from build123d import *

# Parameters (mm, degrees)
BOSS_EXTRUDE2_DEPTH = 33
CUT_EXTRUDE1_DEPTH  = 28
SKETCH3_R           = 10
CUT_EXTRUDE2_DEPTH  = 6
SKETCH5_R           = 2.9
BOSS_EXTRUDE3_DEPTH = 28.7
CIRPATTERN1_COUNT   = 3
SKETCH6_R           = 1
BOSS_EXTRUDE4_DEPTH = 2


with BuildPart() as part:
    # Sketch1 → Boss-Extrude2 (new body)
    with BuildSketch(Plane(origin=(0, 0, 0), x_dir=(1, 0, 0), z_dir=(0, 1, 0))):
        with BuildLine():
            Line((68.783761953, -39.4), (157.583761953, -39.4))
            ThreePointArc((157.583761953, -39.4), (164.654829765, -36.471067812), (167.583761953, -29.4))
            Line((167.583761953, -29.4), (167.583761953, 29.4))
            ThreePointArc((167.583761953, 29.4), (164.654829765, 36.471067812), (157.583761953, 39.4))
            Line((157.583761953, 39.4), (68.783761953, 39.4))
            ThreePointArc((68.783761953, 39.4), (61.283761953, 46.9), (53.783761953, 39.4))
            Line((53.783761953, 39.4), (30.783761953, 39.4))
            ThreePointArc((30.783761953, 39.4), (21.761629353, 45.015902611), (11.75641742, 48.598216525))
            ThreePointArc((11.75641742, 48.598216525), (10.817431593, 49.174777372), (10.394956543, 50.192437248))
            Line((10.394956543, 50.192437248), (8.132117785, 78.35566571))
            ThreePointArc((8.132117785, 78.35566571), (7.562644675, 79.526094921), (6.350366597, 80))
            Line((6.350366597, 80), (-6.350366597, 80))
            ThreePointArc((-6.350366597, 80), (-7.562644675, 79.526094921), (-8.132117785, 78.35566571))
            Line((-8.132117785, 78.35566571), (-10.394956543, 50.192437248))
            ThreePointArc((-10.394956543, 50.192437248), (-10.817431593, 49.174777372), (-11.75641742, 48.598216525))
            ThreePointArc((-11.75641742, 48.598216525), (-50, 0), (-11.75641742, -48.598216525))
            ThreePointArc((-11.75641742, -48.598216525), (-10.817431593, -49.174777372), (-10.394956543, -50.192437248))
            Line((-10.394956543, -50.192437248), (-8.132117785, -78.35566571))
            ThreePointArc((-8.132117785, -78.35566571), (-7.562644675, -79.526094921), (-6.350366597, -80))
            Line((-6.350366597, -80), (6.350366597, -80))
            ThreePointArc((6.350366597, -80), (7.562644675, -79.526094921), (8.132117785, -78.35566571))
            Line((8.132117785, -78.35566571), (10.394956543, -50.192437248))
            ThreePointArc((10.394956543, -50.192437248), (10.817431593, -49.174777372), (11.75641742, -48.598216525))
            ThreePointArc((11.75641742, -48.598216525), (21.761629353, -45.015902611), (30.783761953, -39.4))
            Line((30.783761953, -39.4), (53.783761953, -39.4))
            ThreePointArc((53.783761953, -39.4), (61.283761953, -46.9), (68.783761953, -39.4))
        make_face()
    extrude(amount=BOSS_EXTRUDE2_DEPTH)

    # Sketch2 → Cut-Extrude1 (cut)
    with BuildSketch(Plane(origin=(0, 33, 0), x_dir=(1, 0, 0), z_dir=(0, 1, 0))):
        with BuildLine():
            Line((23.583761953, 29.4), (23.583761953, -29.4))
            ThreePointArc((23.583761953, -29.4), (25.702607781, -35.555274886), (31.161243737, -39.102134069))
            ThreePointArc((31.161243737, -39.102134069), (22.770762082, -44.513957297), (13.472291615, -48.150777342))
            Line((13.472291615, -48.150777342), (13.472291615, -85.250601705))
            Line((13.472291615, -85.250601705), (-13.472291615, -85.250601705))
            Line((-13.472291615, -85.250601705), (-13.472291615, -48.150777342))
            ThreePointArc((-13.472291615, -48.150777342), (-50, 0), (-13.472291615, 48.150777342))
            Line((-13.472291615, 48.150777342), (-13.472291615, 85.250601705))
            Line((-13.472291615, 85.250601705), (13.472291615, 85.250601705))
            Line((13.472291615, 85.250601705), (13.472291615, 48.150777342))
            ThreePointArc((13.472291615, 48.150777342), (22.770762082, 44.513957297), (31.161243737, 39.102134069))
            ThreePointArc((31.161243737, 39.102134069), (25.702607781, 35.555274886), (23.583761953, 29.4))
        make_face()
    extrude(amount=-CUT_EXTRUDE1_DEPTH, mode=Mode.SUBTRACT)

    # Sketch3 → Cut-Extrude2 (cut, through all)
    with BuildSketch(Plane(origin=(0, 5, 0), x_dir=(1, 0, 0), z_dir=(0, 1, 0))):
        Circle(SKETCH3_R)
    extrude(amount=-CUT_EXTRUDE2_DEPTH, mode=Mode.SUBTRACT)

    # Sketch5 → Boss-Extrude3 (add)
    with BuildSketch(Plane(origin=(0, 5, 0), x_dir=(1, 0, 0), z_dir=(0, 1, 0))):
        with Locations((-34.9, 0)):
            Circle(SKETCH5_R)
    boss_extrude3 = extrude(amount=BOSS_EXTRUDE3_DEPTH)

    # CirPattern1: Boss-Extrude3 ×3 about axis
    cirpattern1_axis = Axis((0, 0, 0), (0, 1, 0))
    for i in range(1, CIRPATTERN1_COUNT):
        add(boss_extrude3.rotate(cirpattern1_axis, i * 360 / CIRPATTERN1_COUNT))

    # Sketch6 → Boss-Extrude4 (add)
    with BuildSketch(Plane(origin=(0, 5, 0), x_dir=(1, 0, 0), z_dir=(0, 1, 0))):
        with Locations((-17.896238047, -8.587616886)):
            Circle(SKETCH6_R)
    extrude(amount=BOSS_EXTRUDE4_DEPTH)


solid = part.part
Part model, mm, in its own coordinate system. A direction names the side the tool comes from. Coordinates: 2 decimals unless noted, no trailing zeros. Loops run counter-clockwise (first coordinate to the right, second up) from the corner with the lowest first, then second, coordinate; pieces in that order, holes last. Notation, with made-up numbers: M 38,64 L 84,64 A11 ccw 84,70 Z; hole C 82,-0.5 d7. An arc over 180 degrees is marked long. Use a Markdown table: item, result. Add a question column.
Q1. Which spindle directions (+Z, -Z, +X, -X, +Y, -Y) get a long thin tool onto all of the face, cutting with end or side? Do faces 1 (the cylindrical face through (15.31, 19.15, -32.18)), 2 (the flat face through (95, 33, -1)), 3 (the flat face through (113, 16, 39.4)), 4 (the flat face through (0, 2, 80)), 5 (the flat face through (114, 16, -39.4)). Say none if no direction does.
Q2. Cut at B-B (z = 0). Write the cut outline in (x, y), and give its area (3 significant figures).
Q3. Cut at A-A (x = 0). Write the cut outline in (y, z), and give its area (3 significant figures).
Q4. Cut at C-C (y = 12). Write the cut outline in (x, z).
Q5. Cut at D-D (x = 26.5). Write the cut outline in (y, z).
Q6. Probe L1, parallel to Z at x = 0, y = 2.1; L2, parallel to X at y = 2.8, z = 0; L3, parallel to Z at x = 151, y = 19. List the from-to ranges inside material, lowest first.
Q7. Mould opens along X. For faces 6 (the flat face through (167.584, 16, 0)), 7 (the flat face through (18, 33.7, -30)), 8 (the cylindrical face through (-32.134, 19.149, -0.871)) say: +X half, -X half, draft (parallel to the pull), parting line (faces both ways), or undercut.
Q8. Pin check, flat tips, straight feed: P1, Ø11.5, axis at x = 40.5, y = 24.5, coming from the +Z side; P2, Ø10, axis at y = 19.5, z = 36, coming from the -X side; P3, Ø0.6, axis at x = -18, z = 8, coming from the +Y side; P4, Ø1.5, axis at y = 11.5, z = 49.5, coming from the +X side. Stop position of each tip, or through.
Worked out:
| question | item | result |
|---|---|---|
| 1 | face 1 | +Y |
| 1 | face 2 | +Z, -Z, +X, +Y |
| 1 | face 3 | +Z, +X, +Y, -Y |
| 1 | face 4 | +Z, +X, -X, +Y, -Y |
| 1 | face 5 | -Z, +X, +Y, -Y |
| 2 | outline | M -50,0 L -10,0 L -10,5 L -32,5 L -32,33.7 L -37.8,33.7 L -37.8,5 L -50,5 Z; M 10,0 L 167.58,0 L 167.58,33 L 23.58,33 L 23.58,5 L 10,5 Z |
| 2 | area | 5,190 mm2 |
| 3 | outline | M 0,-80 L 5,-80 L 5,-10 L 0,-10 Z; M 0,10 L 5,10 L 5,80 L 0,80 Z |
| 3 | area | 700 mm2 |
| 4 | outline | C -34.9,0 d5.8; C 17.45,-30.22 d5.8; C 17.45,30.22 d5.8; M 23.58,-29.4 A10 ccw 31.16,-39.1 A50 cw 30.78,-39.4 L 53.78,-39.4 A7.5 ccw 68.78,-39.4 L 157.58,-39.4 A10 ccw 167.58,-29.4 L 167.58,29.4 A10 ccw 157.58,39.4 L 68.78,39.4 A7.5 ccw 53.78,39.4 L 30.78,39.4 A50 cw 31.16,39.1 A10 ccw 23.58,29.4 Z |
| 5 | outline | M 0,-42.4 L 5,-42.4 L 5,-36.46 L 33,-36.46 L 33,36.46 L 5,36.46 L 5,42.4 L 0,42.4 Z |
| 6 | L1 | z = -80 to -10, 10 to 80 |
| 6 | L2 | x = -50 to -10, 10 to 167.58 |
| 6 | L3 | z = -39.4 to 39.4 |
| 7 | face 6 | +X half |
| 7 | face 7 | draft |
| 7 | face 8 | undercut |
| 8 | P1 | stops at z = 39.4 |
| 8 | P2 | stops at x = 14.66 |
| 8 | P3 | stops at y = 7 |
| 8 | P4 | passes through |
